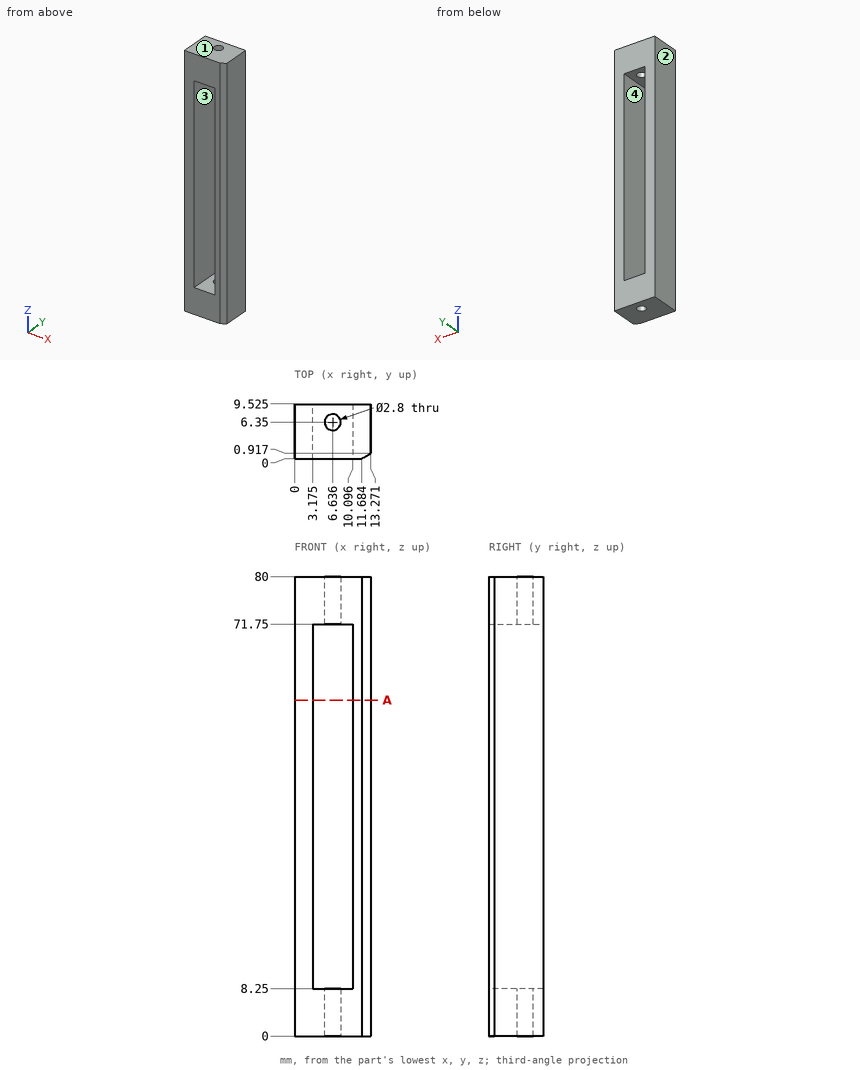
Can you work these out from the drawing? Everything is in mm from the part's minimum corner. Round coordinates to 2 decimals unless told otherwise and drop trailing zeros. Write each loop counter-clockwise with the first axis right and the second up, starting at its lowest first coordinate (ties: lowest second). Pieces come first, ordered by that corner, then holes. Notation, with made-up numbers: (75, 54.5) - (122, 54.5) arc R10 cw to (122, 58.5) - close; hole circle Ø9 at (71, -27.5). An arc over 180 degrees is marked (long way). Put each result on its own line as item: value. Start each with the question number.
(1) I need wall thicknesses on probe 1 along X at (y, z) = (3, 16.5) (1 decimal); probe 2 along Z at (x, y) = (6.5, 1); probe 3 along Y at (x, z) = (12.75, 27) (1 decimal). Which ranges of each line are inside material? Lowest first, please.
(2) Thinking about a two-plate mould opening in X: for the marked faces 1, 2, 3 and 4, which applies, released by +X, released by -X, zero draft, split by the parting line, or undercut?
(3) I want a section at A-A, the plane z = 58.5. Please give me the cut outline in (x, y) (1 decimal).
Here are the results:
1. probe 1: x = 0 to 3.2, 10.1 to 13.3
1. probe 2: z = 0 to 8.25, 71.75 to 80
1. probe 3: y = 0.6 to 9.5
2. face 1: zero draft
2. face 2: released by -X
2. face 3: undercut
2. face 4: undercut
3. outline: (0, 0) - (3.2, 0) - (3.2, 9.5) - (0, 9.5) - close; (10.1, 0) - (11.7, 0) - (13.3, 0.9) - (13.3, 9.5) - (10.1, 9.5) - close
